```python
from build123d import *

# Parameters (mm, degrees)
BOSS_EXTRUDE1_DEPTH       = 9.525
M4_CLEARANCE_HOLE1_D      = 4.5
SKETCH4_R                 = 31.5
CUT_EXTRUDE1_DEPTH        = 68.847075287
M4X0_7_TAPPED_HOLE1_D     = 3.3
M4X0_7_TAPPED_HOLE1_DEPTH = 10
M4X0_7_TAPPED_HOLE1_TIP   = 0.991420021
M4X0_7_TAPPED_HOLE2_D     = 3.3
M4X0_7_TAPPED_HOLE2_DEPTH = 10
M4X0_7_TAPPED_HOLE2_TIP   = 0.991420021


with BuildPart() as part:
    # Sketch1 → Boss-Extrude1 (new body)
    with BuildSketch(Plane.XY):
        with BuildLine():
            Line((-25, 47.5), (25, 47.5))
            Line((25, 47.5), (39.154013015, 26.892624729))
            ThreePointArc((39.154013015, 26.892624729), (47.5, 0), (39.154013015, -26.892624729))
            Line((39.154013015, -26.892624729), (25, -47.5))
            Line((25, -47.5), (-25, -47.5))
            Line((-25, -47.5), (-39.154013015, -26.892624729))
            ThreePointArc((-39.154013015, -26.892624729), (-47.5, 0), (-39.154013015, 26.892624729))
            Line((-39.154013015, 26.892624729), (-25, 47.5))
        make_face()
    extrude(amount=-BOSS_EXTRUDE1_DEPTH)

    # M4 Clearance Hole1 (through all)
    with Locations(Plane.XY):
        with Locations((-30.743901834, 17.75), (0, 35.5), (59.233049824, 29.038488654), (30.743901834, 17.75), (30.743901834, -17.75), (0, -35.5), (-30.743901834, -17.75)):
            Hole(M4_CLEARANCE_HOLE1_D / 2)

    # Sketch4 → Cut-Extrude1 (cut, through all)
    with BuildSketch(Plane(origin=(0, 0, -9.525), x_dir=(-1, 0, 0), z_dir=(0, 0, -1))):
        Circle(SKETCH4_R)
    extrude(amount=-CUT_EXTRUDE1_DEPTH, mode=Mode.SUBTRACT)

    # M4x0.7 Tapped Hole1
    with Locations(Plane(origin=(0, 47.5, 0), x_dir=(1, 0, 0), z_dir=(0, 1, 0))):
        with Locations((16.67, 4.7625), (0, 4.7625), (-16.67, 4.7625)):
            Hole(M4X0_7_TAPPED_HOLE1_D / 2, depth=M4X0_7_TAPPED_HOLE1_DEPTH)
            with Locations((0, 0, -(M4X0_7_TAPPED_HOLE1_DEPTH + M4X0_7_TAPPED_HOLE1_TIP / 2))):  # 118° drill point
                Cone(0, M4X0_7_TAPPED_HOLE1_D / 2, M4X0_7_TAPPED_HOLE1_TIP, mode=Mode.SUBTRACT)

    # M4x0.7 Tapped Hole2
    with Locations(Plane.XZ.offset(47.5)):
        with Locations((0, -4.7625), (16.67, -4.7625), (-16.67, -4.7625)):
            Hole(M4X0_7_TAPPED_HOLE2_D / 2, depth=M4X0_7_TAPPED_HOLE2_DEPTH)
            with Locations((0, 0, -(M4X0_7_TAPPED_HOLE2_DEPTH + M4X0_7_TAPPED_HOLE2_TIP / 2))):  # 118° drill point
                Cone(0, M4X0_7_TAPPED_HOLE2_D / 2, M4X0_7_TAPPED_HOLE2_TIP, mode=Mode.SUBTRACT)


solid = part.part
```
Here's how the part is built. I have some questions about the finished solid (model axes, mm). A direction names the side the tool comes from. Give positions to 0.01 mm unless a question says otherwise; leave off trailing zeros. Order: outer loops, then holes, each group sorted by start corner. A loop starts at its lowest first (then second) coordinate and runs counter-clockwise, first axis right, second up. Notation, with made-up numbers: (-8, 5) - (-2, 5) arc R20 ccw to (-2, 34) - close; hole circle Ø10 at (37, 87.25). An arc over 180 degrees is marked (long way). Answer as a JSON object with one key per item and string values. Group by question number.
Item 1: If we section it at B-B on z = -2: Please give me the cut outline in (x, y).
Item 2: If we mould it in two halves opening along X, with no side actions, what happens to faces 1 (the cylindrical face through (0.358, -42.43, -6.373)), 2 (the cylindrical face through (0.2, 42.4, -6.4)), 3 (the cylindrical face through (-47.5, -0.4, -4.7)), 4 (the flat face through (0, -47.5, -7))? For each: pulls with the +X half, pulls with the -X half, needs draft (parallel to the pull), parting line crosses it, or undercut.
Item 3: If we section it at C-C on x = -19.5: Please give me the cut outline in (y, z) (3 decimals).
Item 4: If we section it at A-A on y = 0: Please give me the cut outline in (x, z) (3 decimals).
Item 5: If we section it at D-D on y = 17.75: Please give me the cut outline in (x, z) (3 decimals).
Item 6: Which directions (+Z, -Z, +X, -X, +Y, -Y) give clear straight access to the entire face, cutting with the end or side of a thin tool? Please do faces 5 (the cylindrical face through (32.53, -19.12, -4.83)), 6 (the cylindrical face through (-17.431, -42.43, -6.226)), 7 (the cylindrical face through (17.886, 42.43, -5.878)).
Item 7: For P1, Ø4.5, axis at x = 0, z = -4.76, coming from the +Y side; P2, Ø1, axis at y = -18.5, z = -6.5, coming from the -X side; P3, Ø3, axis at y = 12.5, z = -6.5, coming from the -X side; P4, Ø2, axis at x = -16.67, z = -4.76, coming from the +Y side, each with a flat end and sliding along its axis, tell me the tip position at first contact or that it passes through.
Item 8: Please list where these lines run through material, in increasing order: probe 1 along Z at (x, y) = (-16.67, -42.5) (1 decimal); probe 2 along X at (y, z) = (17, -2.5); probe 3 along Y at (x, z) = (-1, -9).
Result set:
{
 "1": {"outline": "(-39.15, -26.89) - (-25, -47.5) - (25, -47.5) - (39.15, -26.89) arc R47.5 ccw to (39.15, 26.89) - (25, 47.5) - (-25, 47.5) - (-39.15, 26.89) arc R47.5 ccw to start; hole circle Ø4.5 at (-30.74, -17.75); hole circle Ø4.5 at (-30.74, 17.75); hole circle Ø63 at (0, 0); hole circle Ø4.5 at (0, -35.5); hole circle Ø4.5 at (0, 35.5); hole circle Ø4.5 at (30.74, -17.75); hole circle Ø4.5 at (30.74, 17.75)"},
 "2": {"face 1": "undercut", "face 2": "undercut", "face 3": "pulls with the -X half", "face 4": "needs draft"},
 "3": {"outline": "(-47.5, -9.525) - (-24.739, -9.525) - (-24.739, 0) - (-47.5, 0) - close; (24.739, -9.525) - (47.5, -9.525) - (47.5, 0) - (24.739, 0) - close"},
 "4": {"outline": "(-47.5, -9.525) - (-31.5, -9.525) - (-31.5, 0) - (-47.5, 0) - close; (31.5, -9.525) - (47.5, -9.525) - (47.5, 0) - (31.5, 0) - close"},
 "5": {"outline": "(-44.059, -9.525) - (-32.994, -9.525) - (-32.994, 0) - (-44.059, 0) - close; (-28.494, -9.525) - (-26.023, -9.525) - (-26.023, 0) - (-28.494, 0) - close; (26.023, -9.525) - (28.494, -9.525) - (28.494, 0) - (26.023, 0) - close; (32.994, -9.525) - (44.059, -9.525) - (44.059, 0) - (32.994, 0) - close"},
 "6": {"face 5": "+Z, -Z", "face 6": "-Y", "face 7": "+Y"},
 "7": {"P1": "y = 47.5", "P2": "x = -43.96", "P3": "x = -46.21", "P4": "y = 37.11"},
 "8": {"probe 1": "-9.5 to -6.4, -3.1 to 0", "probe 2": "-44.35 to -32.87, -28.62 to -26.52, 26.52 to 28.62, 32.87 to 44.35", "probe 3": "-47.5 to -37.52, -33.48 to -31.48, 31.48 to 33.48, 37.52 to 47.5"}
}
